Here's how the part is built. I have some questions about the finished solid (model axes, mm). Round coordinates to 2 decimals unless told otherwise and drop trailing zeros. Loops run counter-clockwise (first coordinate to the right, second up) from the corner with the lowest first, then second, coordinate; pieces in that order, holes last. Notation, with made-up numbers: M 69,-1 L 109,-1 A15 ccw 109,27 Z; hole C 52.25,-37.5 d6. An arc over 180 degrees is marked long. Answer as a JSON object with one key per item and string values.
from build123d import *

# Parameters (mm, degrees)
EXTRUDE_THIN1_DEPTH = 3.75
EXTRUDE_THIN2_DEPTH = 3.75
EXTRUDE_THIN3_DEPTH = 3.75


with BuildPart() as part:
    # Sketch1 → Extrude-Thin1 (new body)
    with BuildSketch(Plane.XY):
        with BuildLine():
            Line((73, 62), (73, 54))
            Line((73, 54), (109, 54))
            Line((109, 54), (109, 62))
            ThreePointArc((109, 62), (109.585786438, 63.414213562), (111, 64))
            Line((111, 64), (119, 64))
            Line((119, 64), (119, 100))
            Line((119, 100), (111, 100))
            ThreePointArc((111, 100), (109.585786438, 100.585786438), (109, 102))
            Line((109, 102), (109, 110))
            Line((109, 110), (73, 110))
            Line((73, 110), (73, 102))
            ThreePointArc((73, 102), (72.414213562, 100.585786438), (71, 100))
            Line((71, 100), (63, 100))
            Line((63, 100), (63, 64))
            Line((63, 64), (71, 64))
            ThreePointArc((71, 64), (72.414213562, 63.414213562), (73, 62))
        make_face()
        with BuildLine():
            Line((76, 62), (76, 57))
            Line((76, 57), (106, 57))
            Line((106, 57), (106, 62))
            ThreePointArc((106, 62), (107.464466094, 65.535533906), (111, 67))
            Line((111, 67), (116, 67))
            Line((116, 67), (116, 97))
            Line((116, 97), (111, 97))
            ThreePointArc((111, 97), (107.464466094, 98.464466094), (106, 102))
            Line((106, 102), (106, 107))
            Line((106, 107), (76, 107))
            Line((76, 107), (76, 102))
            ThreePointArc((76, 102), (74.535533906, 98.464466094), (71, 97))
            Line((71, 97), (66, 97))
            Line((66, 97), (66, 67))
            Line((66, 67), (71, 67))
            ThreePointArc((71, 67), (74.535533906, 65.535533906), (76, 62))
        make_face(mode=Mode.SUBTRACT)
    extrude(amount=EXTRUDE_THIN1_DEPTH)

    # Sketch2 → Extrude-Thin2 (add)
    # profile 1 of 2: a face of its own
    with BuildSketch(Plane.XY):
        with BuildLine():
            Line((74, 85), (74, 79))
            ThreePointArc((74, 79), (73.414213562, 77.585786438), (72, 77))
            Line((72, 77), (66, 77))
            Line((66, 77), (66, 87))
            Line((66, 87), (72, 87))
            ThreePointArc((72, 87), (73.414213562, 86.414213562), (74, 85))
        make_face()
        with BuildLine():
            Line((72.6, 85), (72.6, 79))
            ThreePointArc((72.6, 79), (72.424264069, 78.575735931), (72, 78.4))
            Line((72, 78.4), (67.4, 78.4))
            Line((67.4, 78.4), (67.4, 85.6))
            Line((67.4, 85.6), (72, 85.6))
            ThreePointArc((72, 85.6), (72.424264069, 85.424264069), (72.6, 85))
        make_face(mode=Mode.SUBTRACT)
    # profile 2 of 2: a face of its own
    with BuildSketch(Plane.XY):
        with BuildLine():
            Line((108, 79), (108, 85))
            ThreePointArc((108, 85), (108.585786438, 86.414213562), (110, 87))
            Line((110, 87), (116, 87))
            Line((116, 87), (116, 77))
            Line((116, 77), (110, 77))
            ThreePointArc((110, 77), (108.585786438, 77.585786438), (108, 79))
        make_face()
        with BuildLine():
            Line((109.4, 79), (109.4, 85))
            ThreePointArc((109.4, 85), (109.575735931, 85.424264069), (110, 85.6))
            Line((110, 85.6), (114.6, 85.6))
            Line((114.6, 85.6), (114.6, 78.4))
            Line((114.6, 78.4), (110, 78.4))
            ThreePointArc((110, 78.4), (109.575735931, 78.575735931), (109.4, 79))
        make_face(mode=Mode.SUBTRACT)
    extrude(amount=EXTRUDE_THIN2_DEPTH)

    # Sketch3 → Extrude-Thin3 (add)
    # profile 1 of 2: a face of its own
    with BuildSketch(Plane.XY):
        with BuildLine():
            Line((96, 101), (96, 107))
            Line((96, 107), (86, 107))
            Line((86, 107), (86, 101))
            ThreePointArc((86, 101), (86.585786438, 99.585786438), (88, 99))
            Line((88, 99), (94, 99))
            ThreePointArc((94, 99), (95.414213562, 99.585786438), (96, 101))
        make_face()
        with BuildLine():
            Line((94.6, 101), (94.6, 105.6))
            Line((94.6, 105.6), (87.4, 105.6))
            Line((87.4, 105.6), (87.4, 101))
            ThreePointArc((87.4, 101), (87.575735931, 100.575735931), (88, 100.4))
            Line((88, 100.4), (94, 100.4))
            ThreePointArc((94, 100.4), (94.424264069, 100.575735931), (94.6, 101))
        make_face(mode=Mode.SUBTRACT)
    # profile 2 of 2: a face of its own
    with BuildSketch(Plane.XY):
        with BuildLine():
            Line((86, 63), (86, 57))
            Line((86, 57), (96, 57))
            Line((96, 57), (96, 63))
            ThreePointArc((96, 63), (95.414213562, 64.414213562), (94, 65))
            Line((94, 65), (88, 65))
            ThreePointArc((88, 65), (86.585786438, 64.414213562), (86, 63))
        make_face()
        with BuildLine():
            Line((87.4, 63), (87.4, 58.4))
            Line((87.4, 58.4), (94.6, 58.4))
            Line((94.6, 58.4), (94.6, 63))
            ThreePointArc((94.6, 63), (94.424264069, 63.424264069), (94, 63.6))
            Line((94, 63.6), (88, 63.6))
            ThreePointArc((88, 63.6), (87.575735931, 63.424264069), (87.4, 63))
        make_face(mode=Mode.SUBTRACT)
    extrude(amount=EXTRUDE_THIN3_DEPTH)


solid = part.part
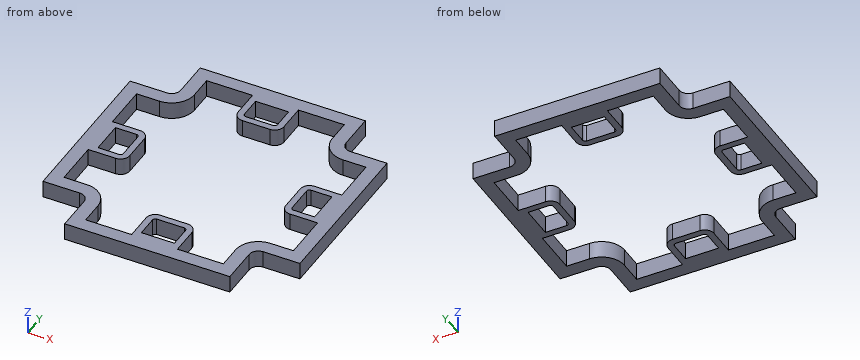
Item 1: I want a section at D-D, the plane y = 95.5. Please give me the cut outline in (x, z), then the cut area to 3 significant figures.
Resolved:
{"outline": "M 63,0 L 66,0 L 66,3.75 L 63,3.75 Z; M 116,0 L 119,0 L 119,3.75 L 116,3.75 Z", "area": "22.5 mm²"}
Item 2: Please list where these lines run through material, in increasing order: probe 1 along Y at (x, z) = (91, 0.95); probe 2 along Y at (x, z) = (111.5, 2.9); probe 3 along Y at (x, z) = (67, 2.55). Write a range as from..to.
Resolved:
{"probe 1": "54..58.4, 63.6..65, 99..100.4, 105.6..110", "probe 2": "64..67, 77..78.4, 85.6..87, 97..100", "probe 3": "64..67, 77..87, 97..100"}
Item 3: I want a section at A-A, the plane x = 107. Please give me the cut outline in (y, z), then the cut area to 3 significant figures.
Resolved:
{"outline": "M 54,0 L 65,0 L 65,3.75 L 54,3.75 Z; M 99,0 L 110,0 L 110,3.75 L 99,3.75 Z", "area": "82.5 mm²"}
Item 4: I want a section at C-C, the plane x = 69.5. Please give me the cut outline in (y, z), then the cut area to 3 significant figures.
Resolved:
{"outline": "M 64,0 L 67,0 L 67,3.75 L 64,3.75 Z; M 77,0 L 78.4,0 L 78.4,3.75 L 77,3.75 Z; M 85.6,0 L 87,0 L 87,3.75 L 85.6,3.75 Z; M 97,0 L 100,0 L 100,3.75 L 97,3.75 Z", "area": "33.0 mm²"}
Item 5: I want a section at B-B, the plane y = 84. Please give me the cut outline in (x, z).
Resolved:
{"outline": "M 63,0 L 67.4,0 L 67.4,3.75 L 63,3.75 Z; M 72.6,0 L 74,0 L 74,3.75 L 72.6,3.75 Z; M 108,0 L 109.4,0 L 109.4,3.75 L 108,3.75 Z; M 114.6,0 L 119,0 L 119,3.75 L 114.6,3.75 Z"}
Item 6: I'm going to push flat-ended pins straight in: pin 1 Ø1.9 at (y, z) = (59, 1.5) entering from +X; pin 2 Ø1.9 at (x, z) = (67.5, 2.5) entering from +Y; pin 3 Ø1.9 at (y, z) = (106, 2) entering from -X. Where does each tip first touch, or does it pass through?
Resolved:
{"pin 1": "x = 109", "pin 2": "y = 100", "pin 3": "x = 73"}
